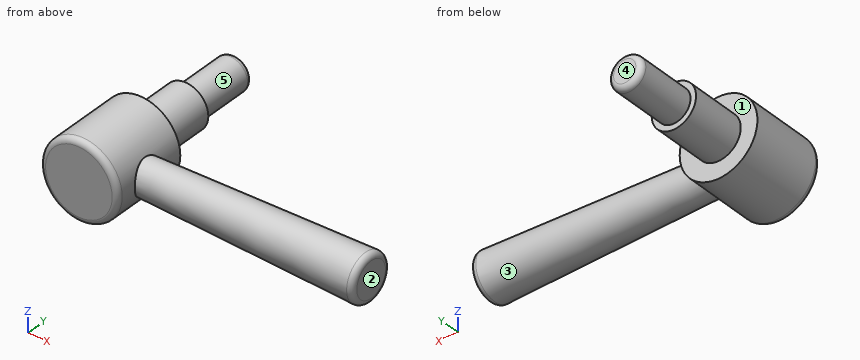
from build123d import *

# Parameters (mm, degrees)
F1_START      = 10
F0_R          = 7
F0_R_2        = 4
F1_DEPTH      = 14
F0_R_3        = 3
F2_DEPTH      = 24
F2_DEPTH_BACK = 11
F3_DEPTH      = 24
F4_R          = 3
F5_DEPTH      = 47
F5_TAPER      = -1.5
F6_R          = 1


with BuildPart() as f1:
    # F0 (on Front) → F1 (new body)
    with BuildSketch(Plane.XZ.offset(F1_START)):
        Circle(F0_R)
        Circle(F0_R_2, mode=Mode.SUBTRACT)
    extrude(amount=F1_DEPTH)



with BuildPart() as f2:
    # F0 (on Front) → F2 (new body, two sides)
    with BuildSketch(Plane.XZ) as f2_sk:
        Circle(F0_R_3)
    extrude(amount=F2_DEPTH)
    extrude(f2_sk.sketch, amount=-F2_DEPTH_BACK)


with BuildPart() as f3:
    # F0 (on Front) → F3 (new body)
    with BuildSketch(Plane.XZ):
        Circle(F0_R_2)
        Circle(F0_R_3, mode=Mode.SUBTRACT)
    extrude(amount=F3_DEPTH)


with BuildPart() as f1_1:
    add(f1.part)

    add(f2.part)  # F5 merges F2

    add(f3.part)  # F5 merges F3
    # F4 (on Right) → F5 (join)
    with BuildSketch(Plane.YZ):
        with Locations((-17, 0)):
            Circle(F4_R)
    extrude(amount=F5_DEPTH, taper=F5_TAPER)

    # F6
    f6_edges = [f1_1.edges().sort_by_distance(p)[0] for p in [
        (-7, -24, 0),
        (47, -21.230738, 0),
        (-3, 11, 0),
    ]]
    fillet(f6_edges, radius=F6_R)


solid = f1_1.part
The model under review builds one solid part; all positions refer to its coordinate system, in mm. Face numbers are marked on the shaded views. A direction names the side the tool comes from. Round coordinates to 2 decimals unless told otherwise and drop trailing zeros. Write each loop counter-clockwise with the first axis right and the second up, starting at its lowest first coordinate (ties: lowest second). Pieces come first, ordered by that corner, then holes. Notation, with made-up numbers: M 27.25,44.25 L 64.25,44.25 A27 cw 64.25,73.25 Z; hole C 57,44 d9. An arc over 180 degrees is marked long. Use a Markdown table: item, result. Add a question column.
Q1. We need section D-D, the plane x = 25. State the section outline as (y, z) points.
Q2. To check wall thickness, follow line 1 (Y direction, x = 16.5, z = 0.75); line 2 (Y direction, x = 25, z = -2); line 3 (Z direction, x = -2, y = -7.5). State the ranges of each line that lie inside material, in increasing order.
Q3. Insertion check: pin 1 (3 mm diameter, centred on y = 4.5, z = -3.5, fed in from +X); pin 2 (8 mm diameter, centred on x = 34.5, z = 4.5, fed in from -Y); pin 3 (5 mm diameter, centred on x = 21, z = 3.5, fed in from +Y). Each pin has a flat end and moves straight along its axis. Give the tip position at first contact, or say it passes through.
Q4. We need section A-A, the plane x = 0. State the section outline as (y, z) points.
Q5. We need section B-B, the plane y = 3. State the section outline as (x, z) points.
Q6. Machinability: for the marked faces 1 and 2, which of the approach directions +Z, -Z, +X, -X, +Y, -Y give a long, thin tool a straight path to every point of the face, cutting with its end or side? Answer none if there is none.
Q7. We need section C-C, the plane y = -17. State the section outline as (x, z) points.
Q8. The part is to be moulded in two halves that separate along X. For the marked faces 3, 4 and 5, say which applies: pulls with the +X half, pulls with the -X half, needs draft (parallel to the pull), parting line crosses it, or undercut.
Findings below:
| question | item | result |
|---|---|---|
| 1 | outline | C -17,0 d7.31 |
| 2 | line 1 | y = -20.35 to -13.65 |
| 2 | line 2 | y = -20.06 to -13.94 |
| 2 | line 3 | z = -3.46 to 3.46 |
| 3 | pin 1 | stops at x = 2.24 |
| 3 | pin 2 | stops at y = -20.88 |
| 3 | pin 3 | stops at y = -13.59 |
| 4 | outline | M -24,-6 A1 ccw -23,-7 L -10,-7 L -10,-4 L 0,-4 L 0,-3 L 10,-3 A1 ccw 11,-2 L 11,2 A1 ccw 10,3 L 0,3 L 0,4 L -10,4 L -10,7 L -23,7 A1 ccw -24,6 Z |
| 5 | outline | C 0,0 d6 |
| 6 | face 1 | +Y |
| 6 | face 2 | +Z, -Z, +X, +Y, -Y |
| 7 | outline | M 6.24,-3.16 L 45.97,-4.2 A1 ccw 47,-3.2 L 47,3.2 A1 ccw 45.97,4.2 L 6.24,3.16 A7 ccw long Z |
| 8 | face 3 | undercut |
| 8 | face 4 | needs draft |
| 8 | face 5 | parting line crosses it |
